Work out the finished part from the listing and answer in its coordinate system (mm). A direction names the side the tool comes from. Give positions to 0.01 mm unless a question says otherwise; leave off trailing zeros. Loops run counter-clockwise (first coordinate to the right, second up) from the corner with the lowest first, then second, coordinate; pieces in that order, holes last. Notation, with made-up numbers: (-27.75, 21) -> (4.25, 21) arc R5 cw to (4.25, 27) -> close; hole circle Ø11 at (19.25, 54.25). An arc over 180 degrees is marked (long way). Answer as CSV lines item,"result". Start each with the question number.
1. A tool of negligible diameter and unlimited length cuts with its end or side. For faces 4 (the face through (13.31, -6.94, 8.99)), 5 (the face through (-6.074, 0.134, -8.125)), 6 (the face through (21, 2.8, 0)), 7 (the face through (0, 0, 0)), from which of +Z, -Z, +X, -X, +Y, -Y can it reach the whole face along a straight path? Write none if from no direction.
2. Find section B-B, the plane x = 9. Give the vertices of the cut face in (y, z).
3. Find section D-D, the plane z = 4.25. Give the vertices of the cut face in (x, y), and give its area (3 significant figures).
4. Determine the mould class of faces 1 (the face through (-6.27, 0.14, -7.68)), 2 (the face through (13.31, 6.96, 9.01)), 3 (the face through (20.986, 1.42, 2.414)) for opening direction X: +X half, -X half, draft (parallel to the pull), parting line (faces both ways), or undercut.
5. Flat-ended cylindrical pins translate along their axes: pin 1 Ø4 at (x, z) = (-4.5, -7.5) entering from -Y; pin 2 Ø2.5 at (y, z) = (0, 0) entering from +X; pin 3 Ø1.5 at (y, z) = (5, -7) entering from -X. Find the tip coordinate at first contact, or state that the pin passes through.
6. Find the intervals of material crossed by line 1 along Z through (x, y) = (14, -4.75); line 2 along Z through (x, y) = (11.5, 6.25); line 3 along X through (y, z) = (-3, -5.25), in increasing order.
7. Find section C-C, the plane x = 15. Give the vertices of the cut face in (y, z), and give its area (3 significant figures).
8. Find section A-A, the plane z = 0. Give the vertices of the cut face in (x, y), and give its area (3 significant figures).
from build123d import *

# Parameters (mm, degrees)
CYLINDER_R           = 7.95
CYLINDER_DEPTH       = 12
PAD_DEPTH            = 27
BOX_W                = 27
BOX_H                = 15.9
BOX_DEPTH            = 12
SKETCH004_W          = 20
SKETCH004_H          = 20
SKETCH004_R          = 3.5
POCKET_DEPTH         = 6
SKETCH005_R          = 3.5
POCKET001_DEPTH      = 5
SKETCH006_R          = 2.5
POCKET002_DEPTH      = 10.001
POCKET002_DEPTH_BACK = 10.001
POCKET003_DEPTH      = 2
SKETCH008_R          = 1.5
POCKET004_DEPTH      = 7.001


with BuildPart() as obj1:
    # Cylinder → Cylinder (new body)
    with BuildSketch(Plane.XY.offset(-6)):
        Circle(CYLINDER_R)
    extrude(amount=CYLINDER_DEPTH)


with BuildPart() as idlerbody:
    # Sketch → Pad (new body)
    with BuildSketch(Plane.YZ):
        Polygon((0, 2), (-7.95, 2), (-5.95, 0), (-7.95, -2), (0, -2), (7.95, -2), (5.95, 0), (7.95, 2), align=None)
    extrude(amount=PAD_DEPTH)

    # Sketch002 (on DatumPlane) → AdditiveLoft section 0
    with BuildSketch(Plane.XY.offset(2)):
        with BuildLine():
            ThreePointArc((0, 7.95), (-7.95, 0), (0, -7.95))
            Line((0, 7.95), (0, -7.95))
        make_face()
    # Sketch001 → AdditiveLoft section 1
    with BuildSketch(Plane.XY):
        with BuildLine():
            ThreePointArc((0, 5.95), (-5.95, 0), (0, -5.95))
            Line((0, 5.95), (0, -5.95))
        make_face()
    # Sketch003 (on DatumPlane) → AdditiveLoft section 2
    with BuildSketch(Plane.XY.offset(-2)):
        with BuildLine():
            ThreePointArc((0, 7.95), (-7.95, 0), (0, -7.95))
            Line((0, 7.95), (0, -7.95))
        make_face()
    loft(ruled=True)


with BuildPart() as idlerbody_1:
    # Body placement: moved
    add(idlerbody.part.moved(Location((0, 0, -8))))


with BuildPart() as idlerbody_mirror:
    # Part__Mirroring: instance of IdlerBody
    add(idlerbody_1.part.mirror(Plane(origin=(0, 0, 0), x_dir=(0, 1, 0), z_dir=(0, 0, 1))))


with BuildPart() as finalcutsbody_refined:
    # Box → Box (new body)
    with BuildSketch(Plane(origin=(0, -7.95, -6), x_dir=(1, 0, 0), z_dir=(0, 0, 1))):
        with Locations((13.5, 7.95)):
            Rectangle(BOX_W, BOX_H)
    extrude(amount=BOX_DEPTH)

    # Fusion: union obj1, IdlerBody_Mirror, IdlerBody
    add(obj1.part)
    add(idlerbody_mirror.part)
    add(idlerbody_1.part)

    # Sketch004 → Pocket (cut, symmetric)
    with BuildSketch(Plane.XY):
        with Locations((10, 0)):
            Rectangle(SKETCH004_W, SKETCH004_H)
        with Locations((9, 0)):
            Circle(SKETCH004_R, mode=Mode.SUBTRACT)
    extrude(amount=POCKET_DEPTH, both=True, mode=Mode.SUBTRACT)

    # Sketch005 → Pocket001 (cut, symmetric)
    with BuildSketch(Plane.XY):
        with Locations((9, 0)):
            Circle(SKETCH005_R)
    extrude(amount=POCKET001_DEPTH, both=True, mode=Mode.SUBTRACT)

    # Sketch006 → Pocket002 (cut, two sides)
    with BuildSketch(Plane.XY) as pocket002_sk:
        with Locations((9, 0)):
            Circle(SKETCH006_R)
    extrude(amount=-POCKET002_DEPTH, mode=Mode.SUBTRACT)
    extrude(pocket002_sk.sketch, amount=POCKET002_DEPTH_BACK, mode=Mode.SUBTRACT)

    # Sketch007 (on DatumPlane) → Pocket003 (cut)
    with BuildSketch(Plane.YZ.offset(20)):
        Polygon((2.8, -1.616581), (2.8, 1.616581), (0, 3.233162), (-2.8, 1.616581), (-2.8, -1.616581), (0, -3.233162), align=None)
    extrude(amount=POCKET003_DEPTH, mode=Mode.SUBTRACT)

    # Sketch008 (on DatumPlane) → Pocket004 (cut, through all)
    with BuildSketch(Plane.YZ.offset(20)):
        Circle(SKETCH008_R)
    extrude(amount=POCKET004_DEPTH, mode=Mode.SUBTRACT)


solid = finalcutsbody_refined.part
Resolved:
1,face 4,"+X, -X, -Y"
1,face 5,"-X"
1,face 6,"none"
1,face 7,"+Y, -Y"
2,outline,"(-7.95, -10) -> (-2.5, -10) -> (-2.5, -5) -> (-3.5, -5) -> (-3.5, -6) -> (-7.95, -6) -> (-5.95, -8) -> close; (-7.95, 6) -> (-3.5, 6) -> (-3.5, 5) -> (-2.5, 5) -> (-2.5, 10) -> (-7.95, 10) -> (-5.95, 8) -> close; (2.5, -10) -> (7.95, -10) -> (5.95, -8) -> (7.95, -6) -> (3.5, -6) -> (3.5, -5) -> (2.5, -5) -> close; (2.5, 5) -> (3.5, 5) -> (3.5, 6) -> (7.95, 6) -> (5.95, 8) -> (7.95, 10) -> (2.5, 10) -> close"
3,outline,"(0, -7.95) -> (0, 7.95) arc R7.95 ccw to start; (20, -7.95) -> (27, -7.95) -> (27, 7.95) -> (20, 7.95) -> close"
3,area,"211 mm^2"
4,face 1,"-X half"
4,face 2,"draft"
4,face 3,"undercut"
5,pin 1,"stops at y = -7.29"
5,pin 2,"stops at x = 0"
5,pin 3,"stops at x = -6.03"
6,line 1,"z = -10 to -6, 6 to 10"
6,line 2,"z = -10 to -8.3, -7.7 to -6, 6 to 7.7, 8.3 to 10"
6,line 3,"x = -7.36 to 0, 7.2 to 10.8, 20 to 27"
7,outline,"(-7.95, -10) -> (7.95, -10) -> (5.95, -8) -> (7.95, -6) -> (-7.95, -6) -> (-5.95, -8) -> close; (-7.95, 6) -> (7.95, 6) -> (5.95, 8) -> (7.95, 10) -> (-7.95, 10) -> (-5.95, 8) -> close"
7,area,"111 mm^2"
8,outline,"(0, -7.95) -> (0, 7.95) arc R7.95 ccw to start; (20, -7.95) -> (27, -7.95) -> (27, -1.5) -> (22, -1.5) -> (22, -2.8) -> (20, -2.8) -> close; (20, 2.8) -> (22, 2.8) -> (22, 1.5) -> (27, 1.5) -> (27, 7.95) -> (20, 7.95) -> close"
8,area,"184 mm^2"
